Autodesk Inventor part; units mm, degrees
ref_plane "Work Plane1" through (0, -8, -48) normal (0, 0, -1) x (0, 1, 0)
ref_plane "Work Plane2" through (0, -8, -48) normal (0, 0, -1) x (0, 1, 0)
ref_plane "YZ Plane" through (0, 0, 0) normal (1, 0, 0) x (0, 1, 0)
sketch "Sketch1" plane through (0, 0, 0) normal (0, 0, 1) x (1, 0, 0)
  circle A0 centre (36, 40) radius 1.7
  line L0 (0, 0) -> (12, 0)
  line L1 (0, 0) -> (0, 384)
  line L2 (12, 384) -> (12, -8)
  circle A1 centre (4, 8) radius 2
  circle A2 centre (36, 24) radius 12
  line L3 (0, 0) -> (60, 0)
  line L4 (60, 0) -> (60, 47.4892)
  line L5 (60, 46) -> (0, 46)
  line L6 (0, 46) -> (0, 0)
  line L7 (0, 4) -> (60, 4)
  circle A3 centre (22.1436, 32) radius 1.7
  circle A4 centre (22.1436, 16) radius 1.7
  circle A5 centre (36, 8) radius 1.7
  circle A6 centre (49.8564, 16) radius 1.7
  circle A7 centre (49.8564, 32) radius 1.7
  circle A8 centre (4, 16) radius 2
  circle A9 centre (4, 24) radius 2
  circle A10 centre (4, 32) radius 2
  circle A11 centre (4, 40) radius 2
  line L8 (22.731, 4) -> (14.2875, 18.6246)
  line L9 (14.2875, 18.6246) -> (12, 18.6246)
  line L10 (36, 0) -> (36, 40) construction
  line L11 (49.269, 4) -> (57.7125, 18.6246)
  line L12 (57.7125, 18.6246) -> (60, 18.6246)
  line L13 (60, 23.7446) -> (12, 23.7446) construction
  line L14 (0, 47.4892) -> (60, 47.4892)
  line L15 (22.731, 43.4892) -> (14.2875, 28.8646)
  line L16 (14.2875, 28.8646) -> (12, 28.8646)
  line L17 (57.7125, 28.8646) -> (60, 28.8646)
  line L18 (49.269, 43.4892) -> (57.7125, 28.8646)
  line L19 (0, 43.4892) -> (12, 43.4892)
  line L20 (22.731, 43.4892) -> (49.269, 43.4892)
  line L21 (60, 28.8646) -> (58.8562, 28.8646)
  line L22 (58.8562, 28.8646) -> (58.8562, 18.6246)
  line L23 (58.8562, 18.6246) -> (60, 18.6246)
  line L24 (60, 18.6246) -> (60, 28.8646)
  line L25 (13.1437, 28.8646) -> (13.1437, 18.6246)
  circle A12 centre (4, 24) radius 3.25
  line L26 (0, 0) -> (60, 0)
  line L27 (60, 0) -> (60, -8)
  line L28 (60, -8) -> (0, -8)
  line L29 (0, -8) -> (0, 0)
  line L30 (0, -4) -> (60, -4)
  circle A13 centre (4, 0) radius 2
  line L31 (41.275, 0) -> (30, 0)
  line L32 (30, 4) -> (30, -4)
  line L33 (30, -4) -> (41.275, -4)
  line L34 (41.275, -4) -> (41.275, 4)
  circle A14 centre (4, 16) radius 3.25
  point P0 (12, 46)
  point P1 (12, 0)
  point P2 (12, 4)
  point P3 (0, 47.4892)
  point P4 (60, 43.4892)
  point P5 (12, 47.4892)
  point P6 (2, 0)
  point P7 (6, 0)
  dimension "d1" = 3.4
  dimension "d2" = 24
  dimension "d7" = 4
  dimension "d8" = 46
  dimension "d9" = 24
  dimension "d10" = 16
  dimension "d13" = 360
  dimension "d15" = 8
  dimension "d16" = 4
  dimension "d17" = 8
  dimension "d20" = 8
  dimension "d34" = 6.5
  dimension "d35" = 8
  dimension "d36" = 4
  dimension "d39" = 6.5
extrude "Extrusion1" add sketch "Sketch1" along normal blind 2.5 contours A13 L0 L1 L7 L2 | A13 L0 | L0 A13 | L0 L2 L30 L29 A13 | L3 L32 L30 L2 | L2 L7 L32 L3 | L7 L1 L19 L2 | L2 L9 L8 L7 | L30 L27 L28 L2 | L2 L28 L29 L30 | L32 L7 L34 L3 | L3 L34 L30 L32 | L2 L16 L25 L9 | L8 L9 L25 L16 L15 L20 L18 L17 L22 L12 L11 L7 | L34 L7 L4 L3 | L3 L27 L30 L34 | L2 L5 L4 L17 L18 L20 L15 L16 | L1 L5 L2 L19 | L1 L14 L2 L5 | L7 L11 L12 L4 | L2 L14 L4 L5 | L12 L22 L17 L4 | A8 | A10 | A14
extrude "Extrusion2" add sketch "Sketch1" against normal blind 2 contours L3 L32 L30 L2 | L2 L7 L32 L3 | L2 L9 L8 L7 | L30 L27 L28 L2 | L32 L7 L34 L3 | L3 L34 L30 L32 | L2 L16 L25 L9 | L8 L9 L25 L16 L15 L20 L18 L17 L22 L12 L11 L7 | L34 L7 L4 L3 | L3 L27 L30 L34 | L2 L5 L4 L17 L18 L20 L15 L16 | L7 L11 L12 L4 | L2 L14 L4 L5 | L12 L22 L17 L4
extrude "Extrusion3" add sketch "Sketch1" against normal blind 65 contours L3 L32 L30 L2 | L2 L7 L32 L3 | L2 L9 L8 L7 | L30 L27 L28 L2 | L3 L34 L30 L32 | L2 L16 L25 L9 | L34 L7 L4 L3 | L3 L27 L30 L34 | L2 L5 L4 L17 L18 L20 L15 L16 | L7 L11 L12 L4 | L2 L14 L4 L5 | L12 L22 L17 L4
sketch "Sketch2" plane through (22.731, 4, -2) normal (0, 1, 0) x (1, 0, 0)
  line L0 (26.5379, 0) -> (0, 0) construction
  line L1 (13.269, 0) -> (12.9065, 63) construction
  line L2 (7.269, 63) -> (18.544, 63) construction
  circle A0 centre (13.1798, 15.5) radius 2.8
  circle A1 centre (12.9957, 47.4995) radius 2.8
  circle A2 centre (29.269, 46.0997) radius 1.55
  circle A3 centre (-2.731, 46.0997) radius 1.55
  point P0 (-22.731, -2)
  point P1 (37.269, 50)
  point P2 (-10.731, 50)
  dimension "d27" = 5.6
  dimension "d28" = 5.6
  dimension "d29" = 32
  dimension "d30" = 63
  dimension "d31" = 15.5
  dimension "d40" = 3.1
  dimension "d41" = 3.1
extrude "Extrusion5" cut sketch "Sketch2" against normal blind 52 contours A0 | A1
extrude "Extrusion6" cut sketch "Sketch2" against normal blind 12 from surface at 43.4892 contours A2 | A3
ref_plane "Work Plane1" through (0, -8, -48) normal (0, 0, -1) x (0, 1, 0)
extrude "Extrusion7" add sketch "Sketch1" against normal blind 4 from surface at -48 contours A13 L0 L1 L7 L2 | A13 L0 | L0 A13 | L0 L2 L30 L29 A13 | L7 L1 L19 L2 | L2 L28 L29 L30 | L1 L5 L2 L19 | L1 L14 L2 L5 | A8 | A10 | A12 | A14
ref_plane "Work Plane2" through (0, -8, -48) normal (0, 0, -1) x (0, 1, 0)
extrude "Extrusion8" cut sketch "Sketch1" against normal blind 0.5 from surface at -48 contours A13 L0 L1 L7 L2 | A13 L0 | L0 A13 | L0 L2 L30 L29 A13 | L7 L1 L19 L2 | L2 L28 L29 L30 | L1 L5 L2 L19 | L1 L14 L2 L5 | A8 | A10 | A12 | A14
equation "\"d31\" = -0.5 * d29 + 0.5 * d30"
equation "\"d41\" = d40"
properties part number "ViperSlide Motor Mount"
Here's how the part is built. I have some questions about the finished solid (model axes, mm). A direction names the side the tool comes from. Round coordinates to 2 decimals unless told otherwise and drop trailing zeros. Loops run counter-clockwise (first coordinate to the right, second up) from the corner with the lowest first, then second, coordinate; pieces in that order, holes last. Notation, with made-up numbers: (1, -33) - (17, -33) arc R13 ccw to (17, -16) - close; hole circle Ø2 at (-34, -26.75). An arc over 180 degrees is marked (long way). One line per question, with ' | ' between items. Start each with the question number.
Q1. I want a section at D-D (z = -17.5). Write out the boundary of the cut face in (x, y) (1 decimal), then the cut area to 3 significant figures.
Q2. For faces 1 (the cylindrical face through (34.65, 9.03, 0.22)), 2 (the flat face through (6, 20, -52)), 3 (the flat face through (0, 19, 1)), 4 (the flat face through (6, 20, 0)), 5 (the flat face through (45, 4, -33)), which set-ups out of +Z, -Z, +X, -X, +Y, -Y let a thin tool reach every point of the face, with its end or its side?
Q3. Will these pins go through, and if not, where does the flat tip stop? pin 1 (13 mm diameter, centred on x = 34, y = 31.5, fed in from -Z); pin 2 (2.5 mm diameter, centred on x = 4, y = 8, fed in from +Z); pin 3 (4 mm diameter, centred on y = 30, z = -57, fed in from -X); pin 4 (13 mm diameter, centred on x = 4.5, y = 30, fed in from -Z).
Q4. I want a section at C-C (z = -36). Write out the boundary of the cut face in (x, y) (1 decimal).
Q5. We'd pull the mould along Z, two halves only. Please class faces 6 (the cylindrical face through (18.45, 43.12, -48.17)), 7 (the flat face through (58.856, 24, -33)), 8 (the flat face through (20, 8, -65)): +Z half, -Z half, draft (parallel to the pull), parting line (faces both ways), or undercut.
Q6. Please list where these lines run through material, in increasing order: line 1 (Y direction, x = 36, z = -0.55); line 2 (Y direction, x = 4, z = -50.3); line 3 (Y direction, x = 25.5, z = -13). Write a range as [from, to].
Q7. I want a section at B-B (x = 4). State how many separate pieces and enclosed holes the cut face has, then the cut area to 3 significant figures.
Q8. I want a section at A-A (y = 24). Write out the boundary of the cut face in (x, z), then the cut area to 3 significant figures.
Response values:
1) outline: (12, -8) - (33.1, -8) - (33.1, 0) - (30, 0) - (30, 4) - (22.7, 4) - (14.3, 18.6) - (13.1, 18.6) - (13.1, 28.9) - (14.3, 28.9) - (22.7, 43.5) - (49.3, 43.5) - (57.7, 28.9) - (58.9, 28.9) - (58.9, 18.6) - (57.7, 18.6) - (49.3, 4) - (41.3, 4) - (41.3, 0) - (38.7, 0) - (38.7, -8) - (60, -8) - (60, 47.5) - (12, 47.5) - close | area: 1,080 mm²
2) face 1: +Z, -Z | face 2: -Z, -X, +Y, -Y | face 3: +Z, -Z, -X, +Y, -Y | face 4: -X, +Y, -Y | face 5: -Z
3) pin 1: stops at z = -2 | pin 2: passes through | pin 3: stops at x = 12 | pin 4: stops at z = -52
4) outline: (12, -8) - (60, -8) - (60, 47.5) - (12, 47.5) - close; hole (13.1, 18.6) - (14.3, 18.6) - (22.7, 4) - (30, 4) - (30, 0) - (41.3, 0) - (41.3, 4) - (49.3, 4) - (57.7, 18.6) - (58.9, 18.6) - (58.9, 28.9) - (57.7, 28.9) - (49.3, 43.5) - (22.7, 43.5) - (14.3, 28.9) - (13.1, 28.9) - close
5) face 6: undercut | face 7: draft | face 8: -Z half
6) line 1: y = [-8, 6.3], [9.7, 12], [36, 38.3], [41.7, 47.49] | line 2: y = [-8, 6], [10, 22], [26, 38], [42, 47.49] | line 3: y = [-8, 4], [43.49, 47.49]
7) separate pieces: 8 | enclosed holes: 0 | area: 255 mm²
8) outline: (0, -52) - (2, -52) - (2, -48.5) - (0, -48.5) - close; (0, 0) - (0.75, 0) - (0.75, 2.5) - (0, 2.5) - close; (6, -52) - (12, -52) - (12, -65) - (13.14, -65) - (13.14, -2) - (24, -2) - (24, 2.5) - (7.25, 2.5) - (7.25, 0) - (12, 0) - (12, -48.5) - (6, -48.5) - close; (48, -2) - (58.86, -2) - (58.86, -65) - (60, -65) - (60, 2.5) - (48, 2.5) - close | area: 294 mm²
